Geometry check sheet. Reference: the model listing, model coordinates, mm. A direction names the side the tool comes from. Give positions to 0.01 mm unless a question says otherwise; leave off trailing zeros. Write each loop counter-clockwise with the first axis right and the second up, starting at its lowest first coordinate (ties: lowest second). Pieces come first, ordered by that corner, then holes. Notation, with made-up numbers: (64, 10.5) - (102, 10.5) arc R24 cw to (102, 40.5) - close; hole circle Ø4 at (85.25, 59.5). An arc over 180 degrees is marked (long way). One line per question, with ' | ' between items. Start each with the question number.
Q1. Release check for a two-part mould opening along Y. For faces 1 (the face through (-11.056, -49.787, 18.093)), 2 (the face through (22, -11, 36.7)), 3 (the face through (-37.377, -28.66, 6.015)) record: +Y half, -Y half, draft (parallel to the pull), parting line (faces both ways), or undercut.
Q2. Gauge pin test, flat ends, axial feed: P1, Ø5, axis at y = 17.5, z = 11.5, coming from the +X side; P2, Ø5, axis at y = 18, z = 23, coming from the +X side; P3, Ø1.5, axis at x = -3.5, y = -38.5, coming from the -Z side. Record the tip position at first contact, or that the pin passes through.
Q3. Set-up check for faces 4 (the face through (-5.051, -22.746, 24.278)), 5 (the face through (10, 22, 12.2)): record each of +Z, -Z, +X, -X, +Y, -Y from which the full face is reachable in a straight line by a thin tool's end or side.
Q4. Section check D-D on y = -25. Record the boundary of the cut face in (x, z).
Q5. Section check C-C on z = 5. Record the boundary of the cut face in (x, y), and give its area (3 significant figures).
Q6. Section check A-A on x = 0. Record the boundary of the cut face in (y, z), and give its area (3 significant figures).
Q7. Thickness scan on L1, parallel to Y at x = 0, z = 21; L2, parallel to Y at x = 0, z = 6.25; L3, parallel to Z at x = 8, y = 37.5. Record the ranges inside material, lowest first. Write a range as [from, to].
```python
from build123d import *

# Parameters (mm, degrees)
F0_R     = 51
F1_DEPTH = 36.7
F2_R     = 47.1
F3_DEPTH = 12.2
F4_R     = 23.3
F5_DEPTH = 85


with BuildPart() as f1:
    # F0 (on Top) → F1 (new body)
    with BuildSketch(Plane.XY):
        Circle(F0_R)
    extrude(amount=F1_DEPTH)

    # F2 (on Top) → F3 (cut)
    with BuildSketch(Plane.XY):
        Circle(F2_R)
    extrude(amount=F3_DEPTH, mode=Mode.SUBTRACT)

    # F4 (on Top) → F5 (cut)
    with BuildSketch(Plane.XY):
        Circle(F4_R)
    extrude(amount=F5_DEPTH, mode=Mode.SUBTRACT)


solid = f1.part
```
Working result:
1) face 1: parting line | face 2: draft | face 3: undercut
2) P1: stops at x = 48.74 | P2: stops at x = 48.59 | P3: stops at z = 12.2
3) face 4: +Z, -Z | face 5: -Z
4) outline: (-44.45, 0) - (-39.92, 0) - (-39.92, 12.2) - (39.92, 12.2) - (39.92, 0) - (44.45, 0) - (44.45, 36.7) - (-44.45, 36.7) - close
5) outline: circle Ø102 at (0, 0); hole circle Ø94.2 at (0, 0) | area: 1,200 mm2
6) outline: (-51, 0) - (-47.1, 0) - (-47.1, 12.2) - (-23.3, 12.2) - (-23.3, 36.7) - (-51, 36.7) - close; (23.3, 12.2) - (47.1, 12.2) - (47.1, 0) - (51, 0) - (51, 36.7) - (23.3, 36.7) - close | area: 1,450 mm2
7) L1: y = [-51, -23.3], [23.3, 51] | L2: y = [-51, -47.1], [47.1, 51] | L3: z = [12.2, 36.7]
